Model file for the job. Use its own axes, mm. A direction names the side the tool comes from. Round coordinates to 2 decimals unless told otherwise and drop trailing zeros. Order: outer loops, then holes, each group sorted by start corner. A loop starts at its lowest first (then second) coordinate and runs counter-clockwise, first axis right, second up. Notation, with made-up numbers: (57.25, -23) - (78.25, -23) arc R19 cw to (78.25, 9) - close; hole circle Ø10 at (61, 58.25). An arc over 180 degrees is marked (long way). Put each result on its own line as item: value. Start each with the question number.
Item 1: Saw through at D-D on z = -2.5. List the corners of the cut face in (x, y).
Item 2: Pin check, flat tip, straight feed: pin 1 Ø0.5 at (x, y) = (-21, 0.5) entering from +Z. Stop position of the tip, or through.
Item 3: Saw through at C-C on x = -18. List the corners of the cut face in (y, z), plus the area to 3 significant figures.
Item 4: Saw through at A-A on z = 7.5. List the corners of the cut face in (x, y), plus the area to 3 significant figures.
Item 5: Mould opens along X. For faces 3 (the face through (-20, 0, 10)), 4 (the face through (0.36, 0.011, -4.304)), 5 (the face through (27.5, 0, 7)) say: pulls with the +X half, pulls with the -X half, needs draft (parallel to the pull), parting line crosses it, or undercut.
Item 6: Probe probe 1 along X at (y, z) = (0.5, 6.75); probe 2 along Z at (x, y) = (0, -0.55); probe 3 along Z at (x, y) = (25.5, -0.05). List the from-to ranges inside material, lowest first.
Item 7: Saw through at B-B on y = -0.5. List the corners of the cut face in (x, z), plus the area to 3 significant figures.
Item 8: Which spindle directions (+Z, -Z, +X, -X, +Y, -Y) get a long thin tool onto all of the face, cutting with end or side? Do faces 1 (the face through (21, 0, 6.076)), 2 (the face through (-26.885, 0.011, 0.397)). Say none if no direction does.
```python
from build123d import *

# Parameters (mm, degrees)
P_IDAT_VYSUNUT_M1_DEPTH       = 0.8
SKICA3_OUTSIDE_W              = 68.578
SKICA3_OUTSIDE_H              = 31.578
ODEBRAT_VYSUNUT_M2_DEPTH      = 31.763317725
SKICA2_W                      = 1.6
SKICA2_H                      = 7.62
ODEBRAT_VYSUNUT_M1_DEPTH      = 31.763317725
ODEBRAT_VYSUNUT_M3_DEPTH      = 31.763317725
ODEBRAT_VYSUNUT_M3_DEPTH_BACK = 31.763317725


with BuildPart() as part:
    # Skica1 → Přidat vysunutím1 (new, symmetric)
    with BuildSketch(Plane(origin=(0, 0, 0), x_dir=(1, 0, 0), z_dir=(0, 1, 0))):
        with BuildLine():
            Line((-27.5, 0), (-27.5, -13.695682438))
            Line((-27.5, -13.695682438), (27.5, -13.695682438))
            Line((27.5, -13.695682438), (27.5, 0))
            ThreePointArc((27.5, 0), (0, 4.304317562), (-27.5, 0))
        make_face()
    extrude(amount=P_IDAT_VYSUNUT_M1_DEPTH, both=True)

    # Skica3 outside → Odebrat vysunutím2 (cut, through all)
    with BuildSketch(Plane(origin=(0, 0.8, 0), x_dir=(1, 0, 0), z_dir=(0, 1, 0))):
        with Locations((0, -4.696)):
            Rectangle(SKICA3_OUTSIDE_W, SKICA3_OUTSIDE_H)
        with BuildLine():
            Line((-27.5, -2.216643209), (-27.5, -10.695682438))
            ThreePointArc((-27.5, -10.695682438), (-26.621320344, -12.817002782), (-24.5, -13.695682438))
            Line((-24.5, -13.695682438), (24.5, -13.695682438))
            ThreePointArc((24.5, -13.695682438), (26.621320344, -12.817002782), (27.5, -10.695682438))
            Line((27.5, -10.695682438), (27.5, -2.216643209))
            ThreePointArc((27.5, -2.216643209), (26.901508151, -0.418655834), (25.344827599, 0.661944349))
            ThreePointArc((25.344827599, 0.661944349), (0, 4.304317562), (-25.344827599, 0.661944349))
            ThreePointArc((-25.344827599, 0.661944349), (-26.901508151, -0.418655834), (-27.5, -2.216643209))
        make_face(mode=Mode.SUBTRACT)
    extrude(amount=-ODEBRAT_VYSUNUT_M2_DEPTH, mode=Mode.SUBTRACT)

    # Skica2 → Odebrat vysunutím1 (cut, through all)
    with BuildSketch(Plane(origin=(0, 0.8, 0), x_dir=(1, 0, 0), z_dir=(0, 1, 0))):
        with Locations((-20.8, -9.885682438)):
            Rectangle(SKICA2_W, SKICA2_H)
        with Locations((20.8, -9.885682438)):
            Rectangle(SKICA2_W, SKICA2_H)
    extrude(amount=-ODEBRAT_VYSUNUT_M1_DEPTH, mode=Mode.SUBTRACT)

    # Skica6 → Odebrat vysunutím3 (cut, two sides: drawn at the far end of the back side and taken through both)
    with BuildSketch(Plane(origin=(0, 0.8, 0), x_dir=(1, 0, 0), z_dir=(0, 1, 0)).offset(-ODEBRAT_VYSUNUT_M3_DEPTH_BACK)):
        with BuildLine():
            Line((-66.724509211, -79.51573971), (-7.429758187, -13.695682438))
            ThreePointArc((-7.429758187, -13.695682438), (0, -10.388865035), (7.429758187, -13.695682438))
            Line((7.429758187, -13.695682438), (66.724509211, -79.51573971))
            Line((66.724509211, -79.51573971), (66.724509211, -256.69528072))
            Line((66.724509211, -256.69528072), (-66.724509211, -256.69528072))
            Line((-66.724509211, -256.69528072), (-66.724509211, -79.51573971))
        make_face()
    extrude(amount=ODEBRAT_VYSUNUT_M3_DEPTH + ODEBRAT_VYSUNUT_M3_DEPTH_BACK, mode=Mode.SUBTRACT)


solid = part.part
```
Results found:
1. outline: (-17.93, -0.8) - (17.93, -0.8) - (17.93, 0.8) - (-17.93, 0.8) - close
2. pin 1: stops at z = 6.08
3. outline: (-0.8, -2.49) - (0.8, -2.49) - (0.8, 13.7) - (-0.8, 13.7) - close
3. area: 25.9 mm²
4. outline: (-27.5, -0.8) - (-21.6, -0.8) - (-21.6, 0.8) - (-27.5, 0.8) - close; (-20, -0.8) - (20, -0.8) - (20, 0.8) - (-20, 0.8) - close; (21.6, -0.8) - (27.5, -0.8) - (27.5, 0.8) - (21.6, 0.8) - close
4. area: 82.9 mm²
5. face 3: undercut
5. face 4: parting line crosses it
5. face 5: pulls with the +X half
6. probe 1: x = -27.5 to -21.6, -20 to 20, 21.6 to 27.5
6. probe 2: z = -4.3 to 10.39
6. probe 3: z = -0.61 to 13.52
7. outline: (-27.5, 2.22) arc R3 ccw to (-25.34, -0.66) arc R90 ccw to (25.34, -0.66) arc R3 ccw to (27.5, 2.22) - (27.5, 10.7) arc R3 ccw to (24.5, 13.7) - (21.6, 13.7) - (21.6, 6.08) - (20, 6.08) - (20, 13.7) - (7.43, 13.7) arc R10 cw to (-7.43, 13.7) - (-20, 13.7) - (-20, 6.08) - (-21.6, 6.08) - (-21.6, 13.7) - (-24.5, 13.7) arc R3 ccw to (-27.5, 10.7) - close
7. area: 848 mm²
8. face 1: +Z, +Y, -Y
8. face 2: -Z, -X, +Y, -Y
